Autodesk Inventor part; units mm, degrees
ref_plane "YZ Plane" through (0, 0, 0) normal (1, 0, 0) x (0, 1, 0)
ref_plane "XZ Plane" through (0, 0, 0) normal (0, 1, 0) x (-1, 0, 0)
ref_plane "XY Plane" through (0, 0, 0) normal (0, 0, 1) x (1, 0, 0)
sketch "Sketch1" plane through (0, 0, 0) normal (0, 0, 1) x (1, 0, 0)
  line L0 (-50, 15) -> (50, 15)
  line L1 (50, 15) -> (50, -15)
  line L2 (50, -15) -> (-50, -15)
  line L3 (-50, -15) -> (-50, 15)
  point P0 (0, 0)
  point P1 (50, 0)
  point P2 (0, 15)
  dimension "d0" = 100
  dimension "d1" = 30
extrude "Extrusion1" add sketch "Sketch1" along normal blind 45
sketch "Sketch2" plane through (0, 0, 45) normal (0, 0, 1) x (1, 0, 0)
  circle A0 centre (0, 0) radius 8
  dimension "d4" = 16
extrude "Extrusion2" cut sketch "Sketch2" against normal through all
properties part number "lead-screw-nut-preview"
Verification items for the finished model (mm, model axes). Give positions to 0.01 mm unless a question says otherwise; leave off trailing zeros. Loops run counter-clockwise (first coordinate to the right, second up) from the corner with the lowest first, then second, coordinate; pieces in that order, holes last.
1. Section check A-A, the plane y = 0. Enter the section's corners in (x, z).
2. Mould release check, pull along X, two halves, no side actions. Record for faces 1 (the cylindrical face through (-1.73, -7.81, 22.82)), 2 (the flat face through (50, 0, 22)), 3 (the flat face through (-50, 0, 22)): released by +X, released by -X, zero draft, split by the parting line, or undercut.
3. Go/stop test with a flat-tipped pin: pin 1 Ø12 at (x, y) = (8, -5) entering from -Z. Record where the tip stops, or that it passes through.
4. Section check C-C, the plane z = 28.5. Enter the section's corners in (x, y), then the cut area to 3 significant figures.
5. Thickness scan on line 1 (Y direction, x = 0, z = 12); line 2 (X direction, y = -5.25, z = 35); line 3 (Y direction, x = -4, z = 9). Record the ranges inside material, lowest first.
6. Section check B-B, the plane x = 0. Enter the section's corners in (y, z).
Geometry says:
1. outline: (-50, 0) - (-8, 0) - (-8, 45) - (-50, 45) - close; (8, 0) - (50, 0) - (50, 45) - (8, 45) - close
2. face 1: undercut
2. face 2: released by +X
2. face 3: released by -X
3. pin 1: stops at z = 0
4. outline: (-50, -15) - (50, -15) - (50, 15) - (-50, 15) - close; hole circle Ø16 at (0, 0)
4. area: 2,800 mm2
5. line 1: y = -15 to -8, 8 to 15
5. line 2: x = -50 to -6.04, 6.04 to 50
5. line 3: y = -15 to -6.93, 6.93 to 15
6. outline: (-15, 0) - (-8, 0) - (-8, 45) - (-15, 45) - close; (8, 0) - (15, 0) - (15, 45) - (8, 45) - close
